Part model, mm, in its own coordinate system. A direction names the side the tool comes from. Coordinates: 2 decimals unless noted, no trailing zeros. Order: outer loops, then holes, each group sorted by start corner. A loop starts at its lowest first (then second) coordinate and runs counter-clockwise, first axis right, second up.
1) Wall check: L1, parallel to Y at x = 40, z = -73; L2, parallel to Z at x = 55.5, y = 0.5; L3, parallel to X at y = 0, z = 70.75. Give the ranges that are in metal, low to high.
2) Cut at D-D (z = -62.5). List the corners of the cut face in (x, y), and give its area (3 significant figures).
3) Cut at B-B (x = 32). List the corners of the cut face in (y, z), and give its area (3 significant figures).
4) Tool access for faces 1 (the cylindrical face through (46, 0, 75)), 2 (the flat face through (30, 0, 60)): list every direction of +Z, -Z, +X, -X, +Y, -Y with a clear straight run to the whole face (end or side of a thin tool).
5) Cut at C-C (x = 40). List the corners of the cut face in (y, z), and give its area (3 significant figures).
6) Mould opens along Z. For faces 3 (the flat face through (60, 0, 75)), 4 (the flat face through (0, 0, 1)), 5 (the flat face through (23, 0, -90)), 6 (the flat face through (22, 0, 90)) say: +Z half, -Z half, draft (parallel to the pull), parting line (faces both ways), or undercut.
7) Cut at A-A (y = 0). List the corners of the cut face in (x, z), and give its area (3 significant figures).
8) Pin check, flat tips, straight feed: pin 1 Ø1.5 at (y, z) = (10, 54.5) entering from +X; pin 2 Ø15.5 at (x, y) = (40, 0) entering from -Z. Stop position of each tip, or through.
```python
from build123d import *

# Parameters (mm, degrees)
SKETCH1_W               = 30
SKETCH1_H               = 40
SKETCH1_W_2             = 120
BOSS_EXTRUDE1_DEPTH     = 15
SKETCH1_3_W             = 30
SKETCH1_3_H             = 40
BOSS_EXTRUDE2_DEPTH     = 60
CUT_EXTRUDE1_DEPTH      = 163.788205961
CUT_EXTRUDE1_DEPTH_BACK = 163.788205961
SKETCH2_R               = 6


with BuildPart() as part:
    # Sketch1 → Boss-Extrude1 (new body)
    with BuildSketch(Plane(origin=(0, 0, 0), x_dir=(0, 0, -1), z_dir=(1, 0, 0))):
        with Locations((-75, 0)):
            Rectangle(SKETCH1_W, SKETCH1_H)
        Rectangle(SKETCH1_W_2, SKETCH1_H)
        with Locations((75, 0)):
            Rectangle(SKETCH1_W, SKETCH1_H)
    extrude(amount=-BOSS_EXTRUDE1_DEPTH)

    # Sketch1_3 → Boss-Extrude2 (add)
    with BuildSketch(Plane(origin=(0, 0, 0), x_dir=(0, 0, -1), z_dir=(1, 0, 0))):
        with Locations((-75, 0)):
            Rectangle(SKETCH1_3_W, SKETCH1_3_H)
        with Locations((75, 0)):
            Rectangle(SKETCH1_3_W, SKETCH1_3_H)
    extrude(amount=BOSS_EXTRUDE2_DEPTH)

    # Sketch2 → Cut-Extrude1 (cut, two sides: drawn at the far end of the back side and taken through both)
    with BuildSketch(Plane(origin=(0, 0, 60), x_dir=(-1, 0, 0), z_dir=(0, 0, -1)).offset(-CUT_EXTRUDE1_DEPTH_BACK)):
        with Locations((-40, 0)):
            Circle(SKETCH2_R)
    extrude(amount=CUT_EXTRUDE1_DEPTH + CUT_EXTRUDE1_DEPTH_BACK, mode=Mode.SUBTRACT)


solid = part.part
```
Geometry check:
1. L1: y = -20 to -6, 6 to 20
1. L2: z = -90 to -60, 60 to 90
1. L3: x = -15 to 34, 46 to 60
2. outline: (-15, -20) - (60, -20) - (60, 20) - (-15, 20) - close; hole circle Ø12 at (40, 0)
2. area: 2,890 mm2
3. outline: (-20, -90) - (20, -90) - (20, -60) - (-20, -60) - close; (-20, 60) - (20, 60) - (20, 90) - (-20, 90) - close
3. area: 2,400 mm2
4. face 1: +Z, -Z
4. face 2: +X, +Y, -Y
5. outline: (-20, -90) - (-6, -90) - (-6, -60) - (-20, -60) - close; (-20, 60) - (-6, 60) - (-6, 90) - (-20, 90) - close; (6, -90) - (20, -90) - (20, -60) - (6, -60) - close; (6, 60) - (20, 60) - (20, 90) - (6, 90) - close
5. area: 1,680 mm2
6. face 3: draft
6. face 4: undercut
6. face 5: -Z half
6. face 6: +Z half
7. outline: (-15, -90) - (34, -90) - (34, -60) - (0, -60) - (0, 60) - (34, 60) - (34, 90) - (-15, 90) - close; (46, -90) - (60, -90) - (60, -60) - (46, -60) - close; (46, 60) - (60, 60) - (60, 90) - (46, 90) - close
7. area: 5,580 mm2
8. pin 1: stops at x = 0
8. pin 2: stops at z = -90
